Work out the finished part from the listing and answer in its coordinate system (mm). Round coordinates to 2 decimals unless told otherwise and drop trailing zeros. Write each loop counter-clockwise with the first axis right and the second up, starting at its lowest first coordinate (ties: lowest second). Pieces come first, ordered by that corner, then holes. Notation, with made-up numbers: (86, 50) -> (109, 50) arc R9 cw to (109, 62) -> close; hole circle Ø7 at (30.25, 59.25). An arc over 180 degrees is marked (long way). One line per item, written item: value.
```python
from build123d import *

# Parameters (mm, degrees)
F1_DEPTH = 25
F2_R     = 4
F3_DEPTH = 25
F4_SIZE  = 40
F5_DEPTH = 25


with BuildPart() as f1:
    # F0 (on Front) → F1 (new body)
    with BuildSketch(Plane.XZ):
        Polygon((0, 400), (0, 0), (400, 0), (400, 400), (300, 800), (300, 1100), (100, 1100), (100, 800), align=None)
    extrude(amount=F1_DEPTH)

    # F2 (on face) → F3 (cut, through all)
    with BuildSketch(Plane.XZ.offset(25)):
        with Locations((80, 150)):
            Circle(F2_R)
        with Locations((320, 150)):
            Circle(F2_R)
        with Locations((200, 1020)):
            Circle(F2_R)
    extrude(amount=-F3_DEPTH, mode=Mode.SUBTRACT)

    # F4
    f4_edges = [f1.edges().sort_by_distance(p)[0] for p in [
        (400, -12.5, 0),
        (0, -12.5, 0),
        (300, -12.5, 1100),
        (100, -12.5, 1100),
    ]]
    chamfer(f4_edges, length=F4_SIZE)

    # F2 (on face) → F5 (cut)
    with BuildSketch(Plane.XZ.offset(25)):
        with Locations((200, 150)):
            Circle(F2_R)
    extrude(amount=-F5_DEPTH, mode=Mode.SUBTRACT)


solid = f1.part
```
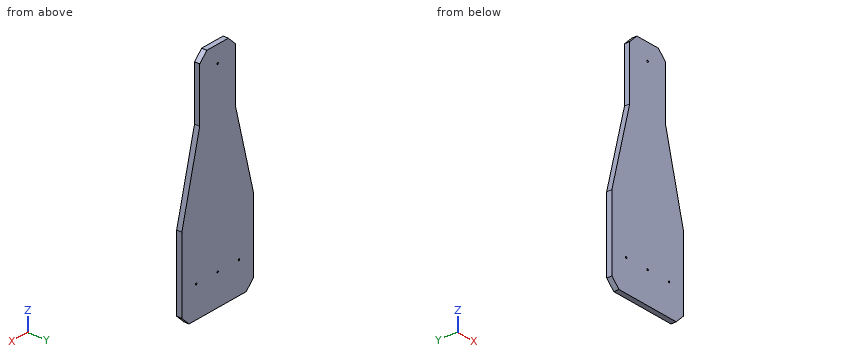
(1) Find section B-B on z = 576. Give the vertices of the cut face in (x, y).
Reported:
outline: (44, -25) -> (356, -25) -> (356, 0) -> (44, 0) -> close
(2) Find section C-C on z = 438.5. Give the vertices of the cut face in (x, y) (3 decimals), plus the area to 3 significant figures.
Reported:
outline: (9.625, -25) -> (390.375, -25) -> (390.375, 0) -> (9.625, 0) -> close
area: 9,520 mm2
(3) A flat-ended cylindrical pin translates along its axis: pin 1 Ø12.5 at (y, z) = (-6.5, 880) entering from -X. Find the tip coordinate at first contact, or state that the pin passes through.
Reported:
pin 1: stops at x = 100
(4) Find section A-A on y = -5.5. Give the vertices of the cut face in (x, z).
Reported:
outline: (0, 40) -> (40, 0) -> (360, 0) -> (400, 40) -> (400, 400) -> (300, 800) -> (300, 1060) -> (260, 1100) -> (140, 1100) -> (100, 1060) -> (100, 800) -> (0, 400) -> close; hole circle Ø8 at (80, 150); hole circle Ø8 at (200, 150); hole circle Ø8 at (200, 1020); hole circle Ø8 at (320, 150)
(5) Consider probe 1 along Z at (x, y) = (200, -7.25); probe 2 along X at (y, z) = (-22.5, 970); probe 3 along X at (y, z) = (-19.5, 1020). Determine where each line is inside the solid, lowest interval first.
Reported:
probe 1: z = 0 to 146, 154 to 1016, 1024 to 1100
probe 2: x = 100 to 300
probe 3: x = 100 to 196, 204 to 300
